Check sheet for the modelled part. Datum: model origin and axes. Units: mm. A direction names the side the tool comes from. Round coordinates to 2 decimals unless told otherwise and drop trailing zeros. Loops run counter-clockwise (first coordinate to the right, second up) from the corner with the lowest first, then second, coordinate; pieces in that order, holes last. Notation, with made-up numbers: (-35, 69) -> (3, 69) arc R16 cw to (3, 74) -> close; hole circle Ø3 at (65, 31.25). An arc over 180 degrees is marked (long way). One line per question, with ' | ' between items.
```python
from build123d import *

# Parameters (mm, degrees)
BOSS_EXTRUDE1_DEPTH     = 2.25
BOSS_EXTRUDE2_DEPTH     = 1.5
CUT_EXTRUDE1_DEPTH      = 4.75
CUT_EXTRUDE1_DEPTH_BACK = 4.75
BOSS_EXTRUDE3_START     = 44.5
SKETCH5_W               = 8
SKETCH5_H               = 12.8
BOSS_EXTRUDE3_DEPTH     = 1.5
BOSS_EXTRUDE4_START     = -44.5
SKETCH5_2_W             = 8
SKETCH5_2_H             = 12.8
BOSS_EXTRUDE4_DEPTH     = 1.5
SKETCH6_R               = 1.2
CUT_EXTRUDE3_DEPTH      = 45.5
CUT_EXTRUDE3_DEPTH_BACK = 45.5
FILLET1_R               = 1.5
SKETCH7_W               = 89
SKETCH7_H               = 89
CUT_EXTRUDE4_DEPTH      = 17.55
SKETCH8_R               = 1.2
BOSS_EXTRUDE5_DEPTH     = 3.75
FILLET2_R               = 1.5


with BuildPart() as part:
    # Sketch1 → Boss-Extrude1 (new body, symmetric)
    with BuildSketch(Plane(origin=(0, 0, 0), x_dir=(1, 0, 0), z_dir=(0, 1, 0))):
        Polygon((-25.5, -35.5), (25.5, -35.5), (35.5, -31.5), (35.5, 31.5), (25.5, 35.5), (-25.5, 35.5), (-35.5, 31.5), (-35.5, -31.5), align=None)
    extrude(amount=BOSS_EXTRUDE1_DEPTH, both=True)

    # Sketch2 → Boss-Extrude2 (add)
    with BuildSketch(Plane(origin=(0, 2.25, 0), x_dir=(1, 0, 0), z_dir=(0, 1, 0))):
        Polygon((27.233241632, -44.5), (44.5, -37.593296653), (44.5, 37.593296653), (27.233241632, 44.5), (-27.233241632, 44.5), (-44.5, 37.593296653), (-44.5, -37.593296653), (-27.233241632, -44.5), align=None)
    boss_extrude2 = extrude(amount=BOSS_EXTRUDE2_DEPTH)

    # Mirror1: Boss-Extrude2 across plane
    add(boss_extrude2.mirror(Plane.ZX))

    # Sketch3 → Cut-Extrude1 (cut, two sides)
    with BuildSketch(Plane(origin=(0, 0, 0), x_dir=(1, 0, 0), z_dir=(0, 1, 0))) as cut_extrude1_sk:
        Polygon((-25.211126395, -34), (25.211126395, -34), (34, -30.484450558), (34, 30.484450558), (25.211126395, 34), (-25.211126395, 34), (-34, 30.484450558), (-34, -30.484450558), align=None)
    extrude(amount=CUT_EXTRUDE1_DEPTH, mode=Mode.SUBTRACT)
    extrude(cut_extrude1_sk.sketch, amount=-CUT_EXTRUDE1_DEPTH_BACK, mode=Mode.SUBTRACT)

    # Sketch5 → Boss-Extrude3 (add)
    with BuildSketch(Plane.XY.offset(BOSS_EXTRUDE3_START)):
        with Locations((-22, 10.15)):
            Rectangle(SKETCH5_W, SKETCH5_H)
        with Locations((22, 10.15)):
            Rectangle(SKETCH5_W, SKETCH5_H)
    extrude(amount=-BOSS_EXTRUDE3_DEPTH)

    # Sketch5<2> → Boss-Extrude4 (add)
    with BuildSketch(Plane.XY.offset(BOSS_EXTRUDE4_START)):
        with Locations((-22, 10.15)):
            Rectangle(SKETCH5_2_W, SKETCH5_2_H)
        with Locations((22, 10.15)):
            Rectangle(SKETCH5_2_W, SKETCH5_2_H)
    extrude(amount=BOSS_EXTRUDE4_DEPTH)

    # Sketch6 → Cut-Extrude3 (cut, two sides)
    with BuildSketch(Plane.XY) as cut_extrude3_sk:
        with Locations((-22, 13.85)):
            Circle(SKETCH6_R)
        with Locations((22, 13.85)):
            Circle(SKETCH6_R)
        with Locations((-22, 8.45)):
            Circle(SKETCH6_R)
        with Locations((22, 8.45)):
            Circle(SKETCH6_R)
    extrude(amount=CUT_EXTRUDE3_DEPTH, mode=Mode.SUBTRACT)
    extrude(cut_extrude3_sk.sketch, amount=-CUT_EXTRUDE3_DEPTH_BACK, mode=Mode.SUBTRACT)

    # Fillet1
    fillet1_edges = [part.edges().sort_by_distance(p)[0] for p in [
        (35.5, 0, 31.5),
        (25.5, 0, 35.5),
        (0, 2.25, -35.5),
        (0, -2.25, -35.5),
        (35.5, 2.25, 0),
        (35.5, -2.25, 0),
        (-35.5, 2.25, 0),
        (-35.5, -2.25, 0),
        (0, 2.25, 35.5),
        (0, -2.25, 35.5),
        (-25.5, 0, -35.5),
        (-30.5, 2.25, -33.5),
        (-35.5, 0, -31.5),
        (-30.5, -2.25, -33.5),
        (35.5, 0, -31.5),
        (30.5, 2.25, -33.5),
        (25.5, 0, -35.5),
        (30.5, -2.25, -33.5),
        (30.5, 2.25, 33.5),
        (30.5, -2.25, 33.5),
        (-35.5, 0, 31.5),
        (-30.5, 2.25, 33.5),
        (-25.5, 0, 35.5),
        (-30.5, -2.25, 33.5),
        (-22, 3.75, -43),
        (22, 3.75, -43),
        (-22, 3.75, 43),
        (22, 3.75, 43),
        (26, 3.75, 43.75),
        (-18, 3.75, 43.75),
        (18, 3.75, 43.75),
        (-26, 3.75, 43.75),
        (18, 3.75, -43.75),
        (26, 3.75, -43.75),
        (-26, 3.75, -43.75),
    ]]
    fillet(fillet1_edges, radius=FILLET1_R)

    # Sketch7 → Cut-Extrude4 (cut, through all)
    with BuildSketch(Plane(origin=(0, 0, 0), x_dir=(1, 0, 0), z_dir=(0, 1, 0))):
        Rectangle(SKETCH7_W, SKETCH7_H)
    extrude(amount=CUT_EXTRUDE4_DEPTH, mode=Mode.SUBTRACT)

    # Sketch8 → Boss-Extrude5 (add)
    with BuildSketch(Plane(origin=(0, 0, 0), x_dir=(1, 0, 0), z_dir=(0, 1, 0))):
        Polygon((34, 30.484450558), (25.211126395, 34), (25.211126395, 27.984450558), (34, 27.984450558), align=None)
        with Locations((27.711126395, 30.484450558)):
            Circle(SKETCH8_R, mode=Mode.SUBTRACT)
        Polygon((-25.211126395, 27.984450558), (-25.211126395, 34), (-34, 30.484450558), (-34, 27.984450558), align=None)
        with Locations((-27.711126395, 30.484450558)):
            Circle(SKETCH8_R, mode=Mode.SUBTRACT)
        Polygon((25.211126395, -27.984450558), (25.211126395, -34), (34, -30.484450558), (34, -27.984450558), align=None)
        with Locations((27.711126395, -30.484450558)):
            Circle(SKETCH8_R, mode=Mode.SUBTRACT)
        Polygon((-34, -30.484450558), (-25.211126395, -34), (-25.211126395, -27.984450558), (-34, -27.984450558), align=None)
        with Locations((-27.711126395, -30.484450558)):
            Circle(SKETCH8_R, mode=Mode.SUBTRACT)
    extrude(amount=-BOSS_EXTRUDE5_DEPTH)

    # Fillet2
    fillet2_edges = [part.edges().sort_by_distance(p)[0] for p in [
        (34, -1.875, -27.984450558),
        (25.211126395, -1.875, -27.984450558),
        (-25.211126395, -1.875, -27.984450558),
        (-34, -1.875, -27.984450558),
        (25.211126395, -1.875, 27.984450558),
        (34, -1.875, 27.984450558),
        (-34, -1.875, 27.984450558),
        (-25.211126395, -1.875, 27.984450558),
        (-25.211126395, -1.875, 34),
        (-25.211126395, -1.875, -34),
        (25.211126395, -1.875, -34),
        (25.211126395, -1.875, 34),
    ]]
    fillet(fillet2_edges, radius=FILLET2_R)


solid = part.part
```
(1) Mould release check, pull along Z, two halves, no side actions. Record for faces 4 (the face through (-35.746, -2.99, -41.095)), 5 (the face through (-34, -2, 0)), 6 (the face through (-30.22, -0.37, 33.61)): +Z half, -Z half, draft (parallel to the pull), parting line (faces both ways), or undercut.
Answer:
face 4: -Z half | face 5: undercut | face 6: +Z half
(2) Set-up check for faces 1 (the face through (25.211, -2, 31)), 2 (the face through (30.22, -0.37, -33.61)), 3 (the face through (-34.4, 0, 2.5)): record each of +Z, -Z, +X, -X, +Y, -Y from which the full face is reachable in a straight line by a thin tool's end or side.
Answer:
face 1: +Y, -Y | face 2: -Z, +X, +Y | face 3: +Z, -Z, +X, -X, +Y
(3) Sectioned sample at B-B, the plane z = -2.5. Record the cut outline in (x, y), and give its area (3 significant figures).
Answer:
outline: (-44.5, -3.75) -> (-34, -3.75) -> (-34, 0) -> (-35.5, 0) -> (-35.5, -0.75) arc R1.5 cw to (-37, -2.25) -> (-44.5, -2.25) -> close; (34, -3.75) -> (44.5, -3.75) -> (44.5, -2.25) -> (37, -2.25) arc R1.5 cw to (35.5, -0.75) -> (35.5, 0) -> (34, 0) -> close | area: 39.2 mm2
(4) Sectioned sample at A-A, the plane x = -8. Record the cut outline in (y, z), and give its area (3 significant figures).
Answer:
outline: (-3.75, -44.5) -> (-2.25, -44.5) -> (-2.25, -37) arc R1.5 cw to (-0.75, -35.5) -> (0, -35.5) -> (0, -34) -> (-3.75, -34) -> close; (-3.75, 34) -> (0, 34) -> (0, 35.5) -> (-0.75, 35.5) arc R1.5 cw to (-2.25, 37) -> (-2.25, 44.5) -> (-3.75, 44.5) -> close | area: 39.2 mm2
(5) Go/stop test with flat-tipped pins: pin 1 (1.1 mm diameter, centred on x = -5, y = -2, fed in from -Z); pin 2 (1.5 mm diameter, centred on x = 4, y = -1, fed in from -Z); pin 3 (1 mm diameter, centred on y = -1, z = 19.5, fed in from +X); pin 4 (1.9 mm diameter, centred on x = 28.5, y = -1, fed in from +Z). Record where each tip stops, or that it passes through.
Answer:
pin 1: stops at z = -44.5 | pin 2: stops at z = -35.88 | pin 3: stops at x = 35.7 | pin 4: stops at z = 35
(6) Scan lines: probe 1 along X at (y, z) = (-2.5, -16); probe 2 along X at (y, z) = (-0.8, -10.5). Record each from-to range of solid material in increasing order.
Answer:
probe 1: x = -44.5 to -34, 34 to 44.5 | probe 2: x = -35.5 to -34, 34 to 35.5
(7) Sectioned sample at C-C, the plane y = -3. Count the separate pieces of the cut face and the enclosed holes in it, and give its area (3 significant figures).
Answer:
separate pieces: 1 | enclosed holes: 5 | area: 3,250 mm2
